Here's the drawing with two shaded views (mm, measured from the low corner). I have some questions. A direction names the side the tool comes from. Coordinates: 2 decimals unless noted, no trailing zeros. Write each loop counter-clockwise with the first axis right and the second up, starting at its lowest first coordinate (ties: lowest second). Pieces come first, ordered by that corner, then holes.
Item 1: Thinking about a two-plate mould opening in Z: for the marked faces 4, 5 and 6, which applies, +Z half, -Z half, draft (parallel to the pull), parting line (faces both ways), or undercut?
Item 2: I want a section at D-D on x = 15.25. Please give me the cut outline in (y, z), then the cut area to 3 significant figures.
Item 3: I want a section at A-A on x = 18. Please give me the cut outline in (y, z).
Item 4: For P1, Ø1, axis at y = 2, z = 4, coming from the +X side; P2, Ø5, axis at y = 6.5, z = 5, coming from the +X side (3 decimals); P3, Ø3, axis at y = 5.5, z = 8.5, coming from the -X side, each with a flat end and sliding along its axis, tell me the tip position at first contact or that it passes through.
Item 5: I want a section at C-C on y = 1.5. Please give me the cut outline in (x, z) (3 decimals).
Item 6: I want a section at B-B on z = 10.5. Please give me the cut outline in (x, y) (3 decimals).
Item 7: If I drill on probe 1 along Y at (x, z) = (11, 9); probe 2 along Z at (x, y) = (6, 11.5); probe 3 along Z at (x, y) = (7.5, 12), over which ranges is the centre line in solid material (lowest first)?
Item 8: Which directions (+Z, -Z, +X, -X, +Y, -Y) give clear straight access to the entire face, cutting with the end or side of a thin tool? Please do the marked faces 1, 2 and 3.
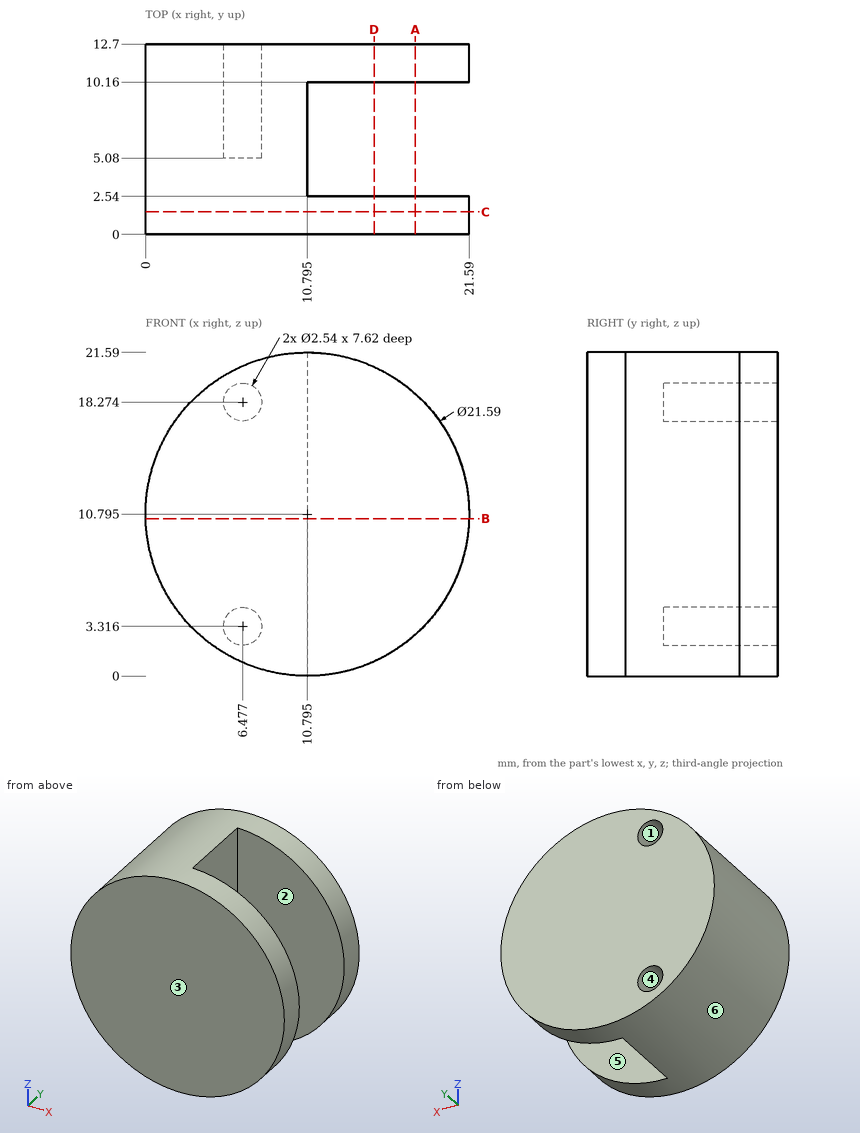
Response values:
1. face 4: undercut
1. face 5: draft
1. face 6: parting line
2. outline: (0, 0.96) - (2.54, 0.96) - (2.54, 20.63) - (0, 20.63) - close; (10.16, 0.96) - (12.7, 0.96) - (12.7, 20.63) - (10.16, 20.63) - close
2. area: 99.9 mm2
3. outline: (0, 2.76) - (2.54, 2.76) - (2.54, 18.83) - (0, 18.83) - close; (10.16, 2.76) - (12.7, 2.76) - (12.7, 18.83) - (10.16, 18.83) - close
4. P1: stops at x = 19.56
4. P2: stops at x = 10.795
4. P3: stops at x = 0.03
5. outline: circle Ø21.59 at (10.795, 10.795)
6. outline: (0.004, 0) - (21.586, 0) - (21.586, 2.54) - (10.795, 2.54) - (10.795, 10.16) - (21.586, 10.16) - (21.586, 12.7) - (0.004, 12.7) - close
7. probe 1: y = 0 to 2.54, 10.16 to 12.7
7. probe 2: z = 1.12 to 2.14, 4.49 to 17.1, 19.45 to 20.47
7. probe 3: z = 0.52 to 2.56, 4.07 to 17.52, 19.03 to 21.07
8. face 1: +Y
8. face 2: +Z, -Z, +X
8. face 3: +Z, -Z, +X, -X, -Y
